```python
from build123d import *

# Parameters (mm, degrees)
SKETCH1_R           = 4
SKETCH1_R_2         = 1.425
BOSS_EXTRUDE1_DEPTH = 61.6
CUT_EXTRUDE1_DEPTH  = 55.6
SKETCH3_R           = 3
SKETCH3_R_2         = 1.55
SKETCH3_R_3         = 1.5
CUT_EXTRUDE2_DEPTH  = 10
SKETCH4_W           = 20.2
SKETCH4_H           = 51.6
SKETCH4_R           = 3
SKETCH4_R_2         = 1.55
SKETCH4_R_3         = 1.5
BOSS_EXTRUDE2_DEPTH = 2
SKETCH5_W           = 15
SKETCH5_H           = 20.2
BOSS_EXTRUDE3_DEPTH = 4
SKETCH6_R           = 1.55
CUT_EXTRUDE3_DEPTH  = 4
FILLET1_R           = 10


with BuildPart() as part:
    # Sketch1 → Boss-Extrude1 (new body)
    with BuildSketch(Plane.XY):
        with BuildLine():
            Line((-10.1, 0), (-10.1, -20))
            Line((-10.1, -20), (10.1, -20))
            Line((10.1, -20), (10.1, 0))
            ThreePointArc((10.1, 0), (0, 10.1), (-10.1, 0))
        make_face()
        with Locations(Location((0, 0, 0), (0, 0, 180))):
            Circle(SKETCH1_R, mode=Mode.SUBTRACT)
        with Locations(Location((0, 7.1, 0), (0, 0, 180))):
            Circle(SKETCH1_R_2, mode=Mode.SUBTRACT)
        with Locations(Location((7.1, 0, 0), (0, 0, 180))):
            Circle(SKETCH1_R_2, mode=Mode.SUBTRACT)
        with Locations(Location((5.020458146, -5.020458146, 0), (0, 0, 180))):
            Circle(SKETCH1_R_2, mode=Mode.SUBTRACT)
        with Locations(Location((0, -7.1, 0), (0, 0, 180))):
            Circle(SKETCH1_R_2, mode=Mode.SUBTRACT)
        with Locations(Location((-5.020458146, -5.020458146, 0), (0, 0, 180))):
            Circle(SKETCH1_R_2, mode=Mode.SUBTRACT)
        with Locations(Location((-7.1, 0, 0), (0, 0, 180))):
            Circle(SKETCH1_R_2, mode=Mode.SUBTRACT)
    extrude(amount=BOSS_EXTRUDE1_DEPTH)

    # Sketch2 → Cut-Extrude1 (cut)
    with BuildSketch(Plane(origin=(10.1, 0, 0), x_dir=(0, 0, -1), z_dir=(1, 0, 0))):
        Polygon((-11.799884689, -18), (-56.6, -18), (-56.6, 10.1), (-5, 10.1), (-5, -18), align=None)
    extrude(amount=-CUT_EXTRUDE1_DEPTH, mode=Mode.SUBTRACT)

    # Sketch3 → Cut-Extrude2 (cut)
    with BuildSketch(Plane.XZ.offset(20)):
        with Locations(Location((0, 30.8, 0), (0, 0, 270))):
            Circle(SKETCH3_R)
        with Locations(Location((-5.084097757, 35.884097757, 0), (0, 0, 270))):
            Circle(SKETCH3_R_2)
        with Locations(Location((5.084097757, 35.884097757, 0), (0, 0, 270))):
            Circle(SKETCH3_R_2)
        with Locations(Location((5.084097757, 25.715902243, 0), (0, 0, 270))):
            Circle(SKETCH3_R_2)
        with Locations(Location((-5.084097757, 25.715902243, 0), (0, 0, 270))):
            Circle(SKETCH3_R_2)
        with Locations(Location((-5.084097757, 46.054097757, 0), (0, 0, 270))):
            Circle(SKETCH3_R_2)
        with Locations(Location((5.084097757, 46.054097757, 0), (0, 0, 270))):
            Circle(SKETCH3_R_2)
        with Locations(Location((-5.084097757, 15.545902243, 0), (0, 0, 270))):
            Circle(SKETCH3_R_3)
        with Locations(Location((5.084097757, 15.545902243, 0), (0, 0, 270))):
            Circle(SKETCH3_R_3)
    extrude(amount=-CUT_EXTRUDE2_DEPTH, mode=Mode.SUBTRACT)

    # Sketch4 → Boss-Extrude2 (add)
    with BuildSketch(Plane(origin=(0, -18, 0), x_dir=(1, 0, 0), z_dir=(0, 1, 0))):
        with Locations((0, -30.8)):
            Rectangle(SKETCH4_W, SKETCH4_H)
        with Locations(Location((0, -30.8, 0), (0, 0, 90))):
            Circle(SKETCH4_R, mode=Mode.SUBTRACT)
        with Locations(Location((-5.084097757, -25.715902243, 0), (0, 0, 90))):
            Circle(SKETCH4_R_2, mode=Mode.SUBTRACT)
        with Locations(Location((5.084097757, -25.715902243, 0), (0, 0, 90))):
            Circle(SKETCH4_R_2, mode=Mode.SUBTRACT)
        with Locations(Location((5.084097757, -15.545902243, 0), (0, 0, 90))):
            Circle(SKETCH4_R_3, mode=Mode.SUBTRACT)
        with Locations(Location((-5.084097757, -15.545902243, 0), (0, 0, 90))):
            Circle(SKETCH4_R_3, mode=Mode.SUBTRACT)
        with Locations(Location((-5.084097757, -35.884097757, 0), (0, 0, 90))):
            Circle(SKETCH4_R_2, mode=Mode.SUBTRACT)
        with Locations(Location((5.084097757, -35.884097757, 0), (0, 0, 90))):
            Circle(SKETCH4_R_2, mode=Mode.SUBTRACT)
        with Locations(Location((-5.084097757, -46.054097757, 0), (0, 0, 90))):
            Circle(SKETCH4_R_2, mode=Mode.SUBTRACT)
        with Locations(Location((5.084097757, -46.054097757, 0), (0, 0, 270))):
            Circle(SKETCH4_R_2, mode=Mode.SUBTRACT)
    extrude(amount=BOSS_EXTRUDE2_DEPTH)

    # Sketch5 → Boss-Extrude3 (add)
    with BuildSketch(Plane(origin=(0, -20, 0), x_dir=(-1, 0, 0), z_dir=(0, -1, 0))):
        with Locations((17.6, -30.8)):
            Rectangle(SKETCH5_W, SKETCH5_H)
        with Locations((-17.6, -30.8)):
            Rectangle(SKETCH5_W, SKETCH5_H)
    extrude(amount=-BOSS_EXTRUDE3_DEPTH)

    # Sketch6 → Cut-Extrude3 (cut)
    with BuildSketch(Plane(origin=(0, -20, 0), x_dir=(-1, 0, 0), z_dir=(0, -1, 0))):
        with Locations(Location((15.254097757, -25.715902243, 0), (0, 0, 90))):
            Circle(SKETCH6_R)
        with Locations(Location((15.254097757, -35.884097757, 0), (0, 0, 270))):
            Circle(SKETCH6_R)
        with Locations(Location((-15.254097757, -25.715902243, 0), (0, 0, 270))):
            Circle(SKETCH6_R)
        with Locations(Location((-15.254097757, -35.884097757, 0), (0, 0, 90))):
            Circle(SKETCH6_R)
    extrude(amount=-CUT_EXTRUDE3_DEPTH, mode=Mode.SUBTRACT)

    # Fillet1
    fillet1_edges = [part.edges().sort_by_distance(p)[0] for p in [
        (-10.1, -18, 20.7),
        (-10.1, -18, 40.9),
        (10.1, -18, 20.7),
        (10.1, -18, 40.9),
    ]]
    fillet(fillet1_edges, radius=FILLET1_R)


solid = part.part
```
Geometry: final body of the model. Coordinates: model frame, mm. A direction names the side the tool comes from. Round coordinates to 2 decimals unless told otherwise and drop trailing zeros. Order: outer loops, then holes, each group sorted by start corner. A loop starts at its lowest first (then second) coordinate and runs counter-clockwise, first axis right, second up. Notation, with made-up numbers: M 59,-14.75 L 81,-14.75 A11 ccw 81,-3.75 Z; hole C 13.5,24 d4. An arc over 180 degrees is marked long. One line per item, written item: value.
(1) Cut plane A-A (z = 30.8). Return the cut outline in (x, y).
Result sheet:
outline: M -25.1,-20 L -3,-20 L -3,-16 L -25.1,-16 Z; M 3,-20 L 25.1,-20 L 25.1,-16 L 3,-16 Z
(2) Pull-direction query (X, two-part tool) for faces 6 (the cylindrical face through (6.15, -4.15, 59.06)), 7 (the flat face through (2, -6, 56.6)), 8 (the flat face through (-25.1, -18, 31)); classes: pulls with the +X half, pulls with the -X half, needs draft (parallel to the pull), parting line crosses it, or undercut.
Result sheet:
face 6: undercut
face 7: needs draft
face 8: pulls with the -X half
(3) Pin query (flat end, axial travel): P1, Ø4, axis at x = -5.08, z = 25.72, coming from the +Y side; P2, Ø1.9, axis at x = -5.08, z = 35.88, coming from the -Y side; P3, Ø3, axis at x = 23, y = -18.5, coming from the +Z side; P4, Ø12, axis at y = -10, z = 6, coming from the +X side. Return the tip coordinate at first contact, or that it passes through.
Result sheet:
P1: y = -16
P2: through
P3: z = 40.9
P4: x = 10.1
(4) Line query: probe 1 along Y at (x, z) = (0, 2) (3 decimals); probe 2 along Z at (x, y) = (-9, -7); probe 3 along X at (y, z) = (-13.5, 57). Output: solid intervals per line, ascending. Write a range as [from, to].
Result sheet:
probe 1: [-20, -8.525], [-5.675, -4], [4, 5.675], [8.525, 10.1]
probe 2: [0, 5], [56.6, 61.6]
probe 3: [-10.1, 10.1]
(5) Reachability of faces 1 (the flat face through (2, -6, 5)), 2 (the flat face through (-10.1, -12, 59)), 3 (the flat face through (10.1, -12, 59)), 4 (the flat face through (-10.1, -12, 3)), 5 (the flat face through (23, -18, 20.7)) from +Z, -Z, +X, -X, +Y, -Y: full face, straight path, thin tool, end or side. Return the list, or none.
Result sheet:
face 1: +X, -X, +Y
face 2: +Z, -X, +Y, -Y
face 3: +Z, +X, +Y, -Y
face 4: -Z, -X, +Y, -Y
face 5: -Z, +X, +Y, -Y
(6) Cut plane C-C (x = 14.5). Return the cut outline in (y, z).
Result sheet:
outline: M -20,18.98 L -16,18.98 L -16,24.36 L -20,24.36 Z; M -20,27.07 L -16,27.07 L -16,34.53 L -20,34.53 Z; M -20,37.24 L -16,37.24 L -16,42.62 L -20,42.62 Z
(7) Cut plane D-D (x = 0). Give the number of separate pieces and of enclosed holes in the cut face, and give its area (3 significant figures).
Result sheet:
separate pieces: 8
enclosed holes: 0
area: 346 mm2
(8) Cut plane B-B (y = 7.1). Return the cut outline in (x, z) (3 decimals).
Result sheet:
outline: M -7.183,0 L -1.425,0 L -1.425,5 L -7.183,5 Z; M -7.183,56.6 L -1.425,56.6 L -1.425,61.6 L -7.183,61.6 Z; M 1.425,0 L 7.183,0 L 7.183,5 L 1.425,5 Z; M 1.425,56.6 L 7.183,56.6 L 7.183,61.6 L 1.425,61.6 Z
